Model file for the job. Use its own axes, mm. A direction names the side the tool comes from. Give positions to 0.01 mm unless a question says otherwise; leave off trailing zeros. Order: outer loops, then holes, each group sorted by start corner. A loop starts at its lowest first (then second) coordinate and runs counter-clockwise, first axis right, second up. Notation, with made-up numbers: (12, -10.75) - (71, -10.75) arc R8 ccw to (71, -1.75) - close; hole circle Ø10 at (-1.5, 5.25). An arc over 180 degrees is marked (long way). Return JSON: item names as keys, results as strings. Group by question number.
from build123d import *

# Parameters (mm, degrees)
F1_DEPTH = 48
F2_W     = 48
F2_H     = 38
F3_DEPTH = 60.001


with BuildPart() as f1:
    # F0 (on Right) → F1 (new body, symmetric)
    with BuildSketch(Plane.YZ):
        with BuildLine():
            ThreePointArc((48, 0), (33.941125, -33.941125), (0, -48))
            Line((0, -48), (0, -72))
            Line((0, -72), (60, -72))
            Line((60, -72), (60, 0))
            Line((60, 0), (48, 0))
        make_face()
    extrude(amount=F1_DEPTH, both=True)

    # F2 (on face) → F3 (cut, through all)
    with BuildSketch(Plane(origin=(0, 60, 0), x_dir=(-1, 0, 0), z_dir=(0, 1, 0))):
        with Locations((0, -19)):
            Rectangle(F2_W, F2_H)
    extrude(amount=-F3_DEPTH, mode=Mode.SUBTRACT)


solid = f1.part
(1) Drop flat-ended pins along their axis: pin 1 Ø4 at (x, y) = (8, 21.5) entering from +Z; pin 2 Ø6 at (x, y) = (-18, 31) entering from +Z; pin 3 Ø3 at (x, z) = (-33.5, -7.5) entering from -Y; pin 4 Ø10 at (y, z) = (40.5, -20) entering from -X. Give the stop position or say it passes through.
(2) Slice it at B-B (z = -16). Give the cut face in (x, y).
(3) 3-axis set-ups, long thin cutter, end or side, ignore diameter. For faces 5 (the face through (0.672, 27.962, -39.014)), 6 (the face through (-24, 52, -23)): which of +Z, -Z, +X, -X, +Y, -Y reach the whole face in a straight line?
(4) Slice it at A-A (y = 54.5). Give the cut face in (x, z), and give its area (3 significant figures).
(5) Slice it at C-C (x = -27). Give the cut face in (y, z), and give its area (3 significant figures).
(6) Drill centre lines: L1, parallel to X at y = 57.5, z = -15; L2, parallel to Z at x = 17, y = 48.5; L3, parallel to Y at x = 34, z = -37. Where is each one in solid material? Low to high.
(7) Pull direction X, two halves, no side cores. Call faces 1 (the face through (48, 36, -43)), 2 (the face through (-48, 36, -43)), 3 (the face through (36, 54, 0)), 4 (the face through (0, 45, -38)): released by +X, released by -X, zero draft, split by the parting line, or undercut.
(8) Slice it at D-D (z = -25). Give the cut face in (x, y).
Result set:
{
 "1": {"pin 1": "stops at z = -41.85", "pin 2": "stops at z = -38", "pin 3": "stops at y = 47.15", "pin 4": "stops at x = -48"},
 "2": {"outline": "(-48, 45.25) - (-24, 45.25) - (-24, 60) - (-48, 60) - close; (24, 45.25) - (48, 45.25) - (48, 60) - (24, 60) - close"},
 "3": {"face 5": "+Z, +X, -X, -Y", "face 6": "+Z, +Y, -Y"},
 "4": {"outline": "(-48, -72) - (48, -72) - (48, 0) - (24, 0) - (24, -38) - (-24, -38) - (-24, 0) - (-48, 0) - close", "area": "5,090 mm²"},
 "5": {"outline": "(0, -72) - (60, -72) - (60, 0) - (48, 0) arc R48 cw to (0, -48) - close", "area": "2,510 mm²"},
 "6": {"L1": "x = -48 to -24, 24 to 48", "L2": "z = -72 to -38", "L3": "y = 30.58 to 60"},
 "7": {"face 1": "released by +X", "face 2": "released by -X", "face 3": "zero draft", "face 4": "undercut"},
 "8": {"outline": "(-48, 40.98) - (-24, 40.98) - (-24, 60) - (-48, 60) - close; (24, 40.98) - (48, 40.98) - (48, 60) - (24, 60) - close"}
}
